Verification items for the finished model (mm, model axes). A direction names the side the tool comes from. Give positions to 0.01 mm unless a question says otherwise; leave off trailing zeros. Write each loop counter-clockwise with the first axis right and the second up, starting at its lowest first coordinate (ties: lowest second). Pieces come first, ordered by that corner, then holes. Notation, with made-up numbers: (39, -23.75) -> (51, -23.75) arc R16 ccw to (51, -17.75) -> close; hole circle Ø11 at (-16.5, 76). An arc over 180 degrees is marked (long way). Use CSV: the item, a comma, the result in double quotes. Start each with the question number.
```python
from build123d import *

# Parameters (mm, degrees)
SKETCH1_W               = 23.1
SKETCH1_H               = 10.8331
BOSS_EXTRUDE1_DEPTH     = 9.9822
SKETCH2_W               = 2.5019
SKETCH2_H               = 0.762
BOSS_EXTRUDE2_DEPTH     = 4.826
SKETCH3_W               = 0.5461
SKETCH3_H               = 0.3937
BOSS_EXTRUDE3_DEPTH     = 5.461
LPATTERN1_COUNT         = 5
LPATTERN1_PITCH         = 2.5654
LPATTERN1_COUNT_DIR2    = 2
LPATTERN1_PITCH_DIR2    = 5.08
SKETCH4_R               = 2.4003
BOSS_EXTRUDE4_DEPTH     = 13.3858
SKETCH5_R               = 1.1303
CUT_EXTRUDE1_DEPTH      = 2.54
SKETCH6_W               = 0.669118354
SKETCH6_H               = 2.7382
CUT_EXTRUDE2_DEPTH      = 1
CUT_EXTRUDE2_DEPTH_BACK = 11.8331


with BuildPart() as part:
    # Sketch1 → Boss-Extrude1 (new body)
    with BuildSketch(Plane(origin=(0, 0, 0), x_dir=(1, 0, 0), z_dir=(0, 1, 0))):
        Rectangle(SKETCH1_W, SKETCH1_H)
    extrude(amount=BOSS_EXTRUDE1_DEPTH)

    # Sketch2 → Boss-Extrude2 (add)
    with BuildSketch(Plane.XZ):
        with Locations((10.29905, -5.03555)):
            Rectangle(SKETCH2_W, SKETCH2_H)
        with Locations((10.29905, 5.03555)):
            Rectangle(SKETCH2_W, SKETCH2_H)
        with Locations((-10.29905, 5.03555)):
            Rectangle(SKETCH2_W, SKETCH2_H)
        with Locations((-10.29905, -5.03555)):
            Rectangle(SKETCH2_W, SKETCH2_H)
    extrude(amount=BOSS_EXTRUDE2_DEPTH)

    # Sketch3 → Boss-Extrude3 (add)
    with BuildSketch(Plane.XZ):
        with Locations((5.26985, -2.5781)):
            Rectangle(SKETCH3_W, SKETCH3_H)
    boss_extrude3 = extrude(amount=BOSS_EXTRUDE3_DEPTH)

    # LPattern1: Boss-Extrude3 5 × 2, 2 skipped
    with Locations(*[(-i * LPATTERN1_PITCH, 0, j * LPATTERN1_PITCH_DIR2) for i in range(LPATTERN1_COUNT) for j in range(LPATTERN1_COUNT_DIR2) if (i, j) not in ((0, 0), (3, 0), (3, 1))]):
        add(boss_extrude3)

    # Sketch4 → Boss-Extrude4 (add)
    with BuildSketch(Plane(origin=(0, 9.9822, 0), x_dir=(1, 0, 0), z_dir=(0, 1, 0))):
        Circle(SKETCH4_R)
    extrude(amount=BOSS_EXTRUDE4_DEPTH)

    # Sketch5 → Cut-Extrude1 (cut)
    with BuildSketch(Plane(origin=(0, 9.9822, 0), x_dir=(1, 0, 0), z_dir=(0, 1, 0))):
        with Locations((9.1186, 0)):
            Circle(SKETCH5_R)
        with Locations((-9.1186, 0)):
            Circle(SKETCH5_R)
    extrude(amount=-CUT_EXTRUDE1_DEPTH, mode=Mode.SUBTRACT)

    # Sketch6 → Cut-Extrude2 (cut, two sides)
    with BuildSketch(Plane(origin=(0, 0, -5.41655), x_dir=(-1, 0, 0), z_dir=(0, 0, -1))) as cut_extrude2_sk:
        with Locations((-11.215440823, -3.4569)):
            Rectangle(SKETCH6_W, SKETCH6_H)
        with Locations((-9.382659177, -3.4569)):
            Rectangle(SKETCH6_W, SKETCH6_H)
        with Locations((9.382659177, -3.4569)):
            Rectangle(SKETCH6_W, SKETCH6_H)
        with Locations((11.215440823, -3.4569)):
            Rectangle(SKETCH6_W, SKETCH6_H)
    extrude(amount=CUT_EXTRUDE2_DEPTH, mode=Mode.SUBTRACT)
    extrude(cut_extrude2_sk.sketch, amount=-CUT_EXTRUDE2_DEPTH_BACK, mode=Mode.SUBTRACT)


solid = part.part
```
(1) Section check A-A on z = 0. Record the cut outline in (x, y).
(2) Go/stop test with flat-tipped pins: pin 1 (5 mm diameter, centred on y = 13, z = 1, fed in from -X); pin 2 (0.8 mm diameter, centred on y = -3.5, z = 5, fed in from -X); pin 3 (0.6 mm diameter, centred on x = -5, y = -2, fed in from -Z); pin 4 (1 mm diameter, centred on x = 8, y = -2, fed in from +Z). Record where each tip stops, or that it passes through.
(3) Set-up check for faces 1 (the face through (-0.31, 16.58, -2.38)), 2 (the face through (0, 4, 5.417)), 3 (the face through (10, -2, -4.655)): record each of +Z, -Z, +X, -X, +Y, -Y from which the full face is reachable in a straight line by a thin tool's end or side.
(4) Thickness scan on line 1 (X direction, y = 8.65, z = 0); line 2 (Y direction, x = 2.5, z = -2); line 3 (Y direction, x = -1.5, z = -0.5). Record the ranges inside material, lowest first. Write a range as from..to.
(5) Section check B-B on y = -0.75. Give the number of separate pieces and of enclosed holes in the cut face, then the cut area to 3 significant figures.
(6) Section check D-D on x = 1.75. Record the cut outline in (y, z).
(7) Draft check along X on faces 4 (the face through (-9, 7.442, 0)), 5 (the face through (11.55, 4, 0)), 6 (the face through (-10, -2, 4.655)). Enter one of: released by +X, released by -X, zero draft, split by the parting line, or undercut.
(8) Section check C-C on y = 15.5. Record the cut outline in (x, z), then the cut area to 3 significant figures.
Data:
1,outline,"(-11.55, 0) -> (11.55, 0) -> (11.55, 9.98) -> (10.25, 9.98) -> (10.25, 7.44) -> (7.99, 7.44) -> (7.99, 9.98) -> (2.4, 9.98) -> (2.4, 23.37) -> (-2.4, 23.37) -> (-2.4, 9.98) -> (-7.99, 9.98) -> (-7.99, 7.44) -> (-10.25, 7.44) -> (-10.25, 9.98) -> (-11.55, 9.98) -> close"
2,pin 1,"stops at x = -2.4"
2,pin 2,"stops at x = -10.88"
2,pin 3,"stops at z = -2.77"
2,pin 4,"passes through"
3,face 1,"+Y"
3,face 2,"+Z, +X, -X, +Y, -Y"
3,face 3,"+X, -X, -Y"
4,line 1,"x = -11.55..-10.25, -7.99..7.99, 10.25..11.55"
4,line 2,"y = 0..9.98"
4,line 3,"y = 0..23.37"
5,separate pieces,"12"
5,enclosed holes,"0"
5,area,"9.35 mm2"
6,outline,"(0, -5.42) -> (9.98, -5.42) -> (9.98, -1.64) -> (23.37, -1.64) -> (23.37, 1.64) -> (9.98, 1.64) -> (9.98, 5.42) -> (0, 5.42) -> close"
7,face 4,"undercut"
7,face 5,"released by +X"
7,face 6,"zero draft"
8,outline,"circle Ø4.8 at (0, 0)"
8,area,"18.1 mm2"
